Input: part model. Units: mm. Frame: model coordinates. A direction names the side the tool comes from. Coordinates: 2 decimals unless noted, no trailing zeros. Write each loop counter-clockwise with the first axis right and the second up, starting at its lowest first coordinate (ties: lowest second). Pieces come first, ordered by that corner, then holes. Notation, with made-up numbers: (-33.75, -15) - (6.25, -15) arc R22 ccw to (6.25, 8) - close; hole circle Ø2 at (43.5, -19.75). An arc over 180 degrees is marked (long way). Use a Markdown table: item, result. Add a question column.
Q1. Section query A-A (z = 75). Return the cut outline in (x, y), then the cut area to 3 significant figures.
Q2. Material intervals for probe 1 along Y at (x, z) = (7, 75); probe 2 along X at (y, z) = (67.5, 131.5); probe 3 along Z at (x, y) = (0.25, 110), sorted ascending. Write a range as from..to.
Q3. Set-up query: faces 1 (the face through (-0.18, 69.15, 112.15)), 2 (the face through (-33, 11, 142.5)), 3 (the face through (-33, 11, 157.5)), 4 (the face through (41, 15, 7.5)), 5 (the face through (0, 122.5, 75)). Return all of +Z, -Z, +X, -X, +Y, -Y with unobstructed straight access to the full face (end or side cutting, diameter ignored); none if empty.
Q4. Section query C-C (z = -1). Return the cut outline in (x, y).
Q5. Mould query, pull axis Z, two halves, no side actions, for faces 6 (the face through (41, 15, 157.5)), 7 (the face through (-48.7, 20.3, -0.1)), 8 (the face through (0, 20, 140)). Classes: released by +Z, released by -Z, zero draft, split by the parting line, or undercut.
Q6. Section query D-D (y = 11.5). Return the cut outline in (x, z).
Q7. Pin query (flat end, axial travel): P1, Ø20, axis at x = -40, y = 15, coming from the +Z side; P2, Ø4, axis at y = 72.5, z = 34.5, coming from the -X side; P3, Ø1.5, axis at x = 10.5, z = 33, coming from the -Y side. Return the tip coordinate at first contact, or that it passes through.
Q8. Section query B-B (x = -19). Return the cut outline in (y, z).
from build123d import *

# Parameters (mm, degrees)
SKETCH2_W                = 25
SKETCH2_H                = 5
SKETCH2_H_2              = 15
SKETCH2_W_2              = 73.5
BOSS_EXTRUDE3_DEPTH      = 40
CUT_EXTRUDE1_DEPTH       = 15
CUT_EXTRUDE3_DEPTH       = 25
SKETCH5_W                = 25
SKETCH5_H                = 25
SKETCH5_R                = 7.5
BOSS_EXTRUDE4_DEPTH      = 12.5
BOSS_EXTRUDE4_DEPTH_BACK = 12.5
BOSS_EXTRUDE5_START      = -12.5
BOSS_EXTRUDE5_DEPTH      = 25


with BuildPart() as part:
    # Sketch2 → Boss-Extrude3 (new body)
    with BuildSketch(Plane(origin=(0, 0, 0), x_dir=(1, 0, 0), z_dir=(0, 1, 0))):
        with Locations((0, -10)):
            Rectangle(SKETCH2_W, SKETCH2_H)
        Rectangle(SKETCH2_W, SKETCH2_H_2)
        with Locations((0, 10)):
            Rectangle(SKETCH2_W, SKETCH2_H)
        with Locations((-49.25, 0)):
            Rectangle(SKETCH2_W_2, SKETCH2_H_2)
        with Locations((49.25, 0)):
            Rectangle(SKETCH2_W_2, SKETCH2_H_2)
    extrude(amount=BOSS_EXTRUDE3_DEPTH)

    # Sketch6 → Cut-Extrude1 (cut)
    with BuildSketch(Plane(origin=(0, 0, -7.5), x_dir=(-1, 0, 0), z_dir=(0, 0, -1))):
        Polygon((12.5, 40), (86, 0), (86, 40), align=None)
    cut_extrude1 = extrude(amount=-CUT_EXTRUDE1_DEPTH, mode=Mode.SUBTRACT)

    # Mirror1: Cut-Extrude1 across plane
    add(cut_extrude1.mirror(Plane(origin=(0, 0, 0), x_dir=(0, 0, 1), z_dir=(1, 0, 0))), mode=Mode.SUBTRACT)

    # Sketch7 → Cut-Extrude3 (cut)
    with BuildSketch(Plane.ZY.offset(12.5)):
        Polygon((-12.5, 40), (-7.5, 0), (-12.5, 0), align=None)
    cut_extrude3 = extrude(amount=-CUT_EXTRUDE3_DEPTH, mode=Mode.SUBTRACT)

    # Mirror2: Cut-Extrude3 across plane
    add(cut_extrude3.mirror(Plane.XY), mode=Mode.SUBTRACT)



with BuildPart() as body_2:
    # Sketch5 → Boss-Extrude4 (new body, two sides)
    with BuildSketch(Plane(origin=(0, 0, 0), x_dir=(0, 0, -1), z_dir=(1, 0, 0))) as boss_extrude4_sk:
        with Locations((-75, 110)):
            Rectangle(SKETCH5_W, SKETCH5_H)
        with Locations((-75, 110)):
            Circle(SKETCH5_R, mode=Mode.SUBTRACT)
    extrude(amount=BOSS_EXTRUDE4_DEPTH)
    extrude(boss_extrude4_sk.sketch, amount=-BOSS_EXTRUDE4_DEPTH_BACK)


with BuildPart() as part_1:
    add(part.part)

    add(body_2.part)  # Boss-Extrude5 merges body 2
    # Sketch8 → Boss-Extrude5 (add)
    with BuildSketch(Plane(origin=(0, 0, 0), x_dir=(0, 0, -1), z_dir=(1, 0, 0)).offset(BOSS_EXTRUDE5_START)):
        Polygon((-62.5, 97.5), (-12.5, 40), (12.5, 40), (-62.5, 122.5), align=None)
    extrude(amount=BOSS_EXTRUDE5_DEPTH)

    # Mirror13: part across plane


with BuildPart() as part_2:
    add(part_1.part)
    add(part_1.part.mirror(Plane.XY.offset(75)))


solid = part_2.part
Values follow:
| question | item | result |
|---|---|---|
| 1 | outline | (-12.5, 97.5) - (12.5, 97.5) - (12.5, 102.5) - (-12.5, 102.5) - close; (-12.5, 117.5) - (12.5, 117.5) - (12.5, 122.5) - (-12.5, 122.5) - close |
| 1 | area | 250 mm2 |
| 2 | probe 1 | 97.5..102.5, 117.5..122.5 |
| 2 | probe 2 | -12.5..12.5 |
| 2 | probe 3 | 51.14..67.5, 82.5..98.86 |
| 3 | face 1 | +X, -X, -Y |
| 3 | face 2 | -X, +Y, -Y |
| 3 | face 3 | +Z, -X, +Y, -Y |
| 3 | face 4 | +X, +Y, -Y |
| 3 | face 5 | +Z, -Z, +X, -X, +Y |
| 4 | outline | (-86, 0) - (86, 0) - (12.5, 40) - (12.5, 52.65) - (-12.5, 52.65) - (-12.5, 40) - close |
| 5 | face 6 | released by +Z |
| 5 | face 7 | zero draft |
| 5 | face 8 | undercut |
| 6 | outline | (-64.87, -7.5) - (-12.5, -7.5) - (-12.5, -8.94) - (12.5, -8.94) - (12.5, -7.5) - (64.87, -7.5) - (64.87, 7.5) - (12.5, 7.5) - (12.5, 8.94) - (-12.5, 8.94) - (-12.5, 7.5) - (-64.87, 7.5) - close; (-64.87, 142.5) - (-12.5, 142.5) - (-12.5, 141.06) - (12.5, 141.06) - (12.5, 142.5) - (64.87, 142.5) - (64.87, 157.5) - (12.5, 157.5) - (12.5, 158.94) - (-12.5, 158.94) - (-12.5, 157.5) - (-64.87, 157.5) - close |
| 7 | P1 | z = 157.5 |
| 7 | P2 | x = -12.5 |
| 7 | P3 | y = 62.71 |
| 8 | outline | (0, -7.5) - (36.46, -7.5) - (36.46, 7.5) - (0, 7.5) - close; (0, 142.5) - (36.46, 142.5) - (36.46, 157.5) - (0, 157.5) - close |
